Can you work these out from the model? Positions are in its coordinate system, mm. Face numbers are marked on the shaded views. A direction names the side the tool comes from. Give positions to 0.01 mm unless a question says otherwise; leave off trailing zeros. Loops run counter-clockwise (first coordinate to the right, second up) from the corner with the lowest first, then second, coordinate; pieces in that order, holes last. Notation, with made-up numbers: M 37,18.25 L 48,18.25 A28 ccw 48,41.25 Z; hole C 48,-22.5 d4. An arc over 180 degrees is marked long. Use CSV: the item, a comma, the result in double quotes.
from build123d import *

# Parameters (mm, degrees)
RESSALTO_EXTRUS_O1_DEPTH = 22.5
CHANFRO1_SIZE            = 10
CORTE_EXTRUS_O1_REACH    = 324.073
ESBO_O3_W                = 1139.230904301
ESBO_O3_H                = 709.798033895
CORTE_EXTRUS_O5_DEPTH    = 1.5
ESBO_O5_R                = 3
CORTE_EXTRUS_O6_DEPTH    = 322.972048476
CORTE_EXTRUS_O8_DEPTH    = 10


with BuildPart() as part:
    # Esboço1 → Ressalto-extrusão1 (new, symmetric)
    with BuildSketch(Plane.XY):
        with BuildLine():
            Line((-70, 0), (70, 0))
            ThreePointArc((70, 0), (77.071067812, 2.928932188), (80, 10))
            Line((80, 10), (80, 100))
            ThreePointArc((80, 100), (80.93692213, 104.226182617), (83.572123903, 107.660444431))
            Line((83.572123903, 107.660444431), (111.427876097, 131.034195823))
            ThreePointArc((111.427876097, 131.034195823), (114.06307787, 134.468457637), (115, 138.694640254))
            Line((115, 138.694640254), (115, 290))
            ThreePointArc((115, 290), (112.071067812, 297.071067812), (105, 300))
            Line((105, 300), (-105, 300))
            ThreePointArc((-105, 300), (-112.071067812, 297.071067812), (-115, 290))
            Line((-115, 290), (-115, 138.694640254))
            ThreePointArc((-115, 138.694640254), (-114.06307787, 134.468457637), (-111.427876097, 131.034195823))
            Line((-111.427876097, 131.034195823), (-83.572123903, 107.660444431))
            ThreePointArc((-83.572123903, 107.660444431), (-80.93692213, 104.226182617), (-80, 100))
            Line((-80, 100), (-80, 10))
            ThreePointArc((-80, 10), (-77.071067812, 2.928932188), (-70, 0))
        make_face()
        Polygon((-55, 20), (55, 20), (55, 109.793731589), (90, 139.16221868), (90, 280), (-90, 280), (-90, 139.16221868), (-55, 109.793731589), align=None, mode=Mode.SUBTRACT)
    extrude(amount=RESSALTO_EXTRUS_O1_DEPTH, both=True)

    # Chanfro1
    chanfro1_edges = [part.edges().sort_by_distance(p)[0] for p in [
        (114.06307787, 134.468457637, 22.5),
        (115, 214.347320127, 22.5),
        (115, 214.347320127, -22.5),
        (114.06307787, 134.468457637, -22.5),
        (97.5, 119.347320127, -22.5),
        (80.93692213, 104.226182617, -22.5),
        (80, 55, -22.5),
        (77.071067812, 2.928932188, -22.5),
        (0, 0, -22.5),
        (-77.071067812, 2.928932188, -22.5),
        (-80, 55, -22.5),
        (-80.93692213, 104.226182617, -22.5),
        (-97.5, 119.347320127, -22.5),
        (-114.06307787, 134.468457637, -22.5),
        (-115, 214.347320127, -22.5),
        (-112.071067812, 297.071067812, -22.5),
        (0, 300, -22.5),
        (112.071067812, 297.071067812, -22.5),
        (112.071067812, 297.071067812, 22.5),
        (0, 300, 22.5),
        (-112.071067812, 297.071067812, 22.5),
        (-115, 214.347320127, 22.5),
        (-114.06307787, 134.468457637, 22.5),
        (-97.5, 119.347320127, 22.5),
        (-80.93692213, 104.226182617, 22.5),
        (-80, 55, 22.5),
        (-77.071067812, 2.928932188, 22.5),
        (0, 0, 22.5),
        (77.071067812, 2.928932188, 22.5),
        (80, 55, 22.5),
        (80.93692213, 104.226182617, 22.5),
        (97.5, 119.347320127, 22.5),
    ]]
    chamfer(chanfro1_edges, length=CHANFRO1_SIZE - 0.0001)  # a hair under: the kernel refuses the full size

    # Esboço3 → Corte-extrusão1 (cut, up to next)
    with BuildSketch(Plane.XY, mode=Mode.PRIVATE) as corte_extrus_o1_sk1:
        with Locations((-153.157436203, 152.53565808)):
            Rectangle(ESBO_O3_W, ESBO_O3_H)
    corte_extrus_o1_tool1 = extrude(corte_extrus_o1_sk1.sketch, amount=-CORTE_EXTRUS_O1_REACH, mode=Mode.PRIVATE) & part.part
    add(corte_extrus_o1_tool1.solids().sort_by_distance((-153.157436, 152.535658, 0))[0], mode=Mode.SUBTRACT)

    # Esboço4 → Corte-extrusão5 (cut)
    with BuildSketch(Plane.XY.offset(22.5)):
        Polygon((104, 289), (-104, 289), (-104, 139.160947912), (-69, 109.792460821), (-69, 11), (69, 11), (69, 109.792460821), (104, 139.160947912), align=None)
        Polygon((-90, 280), (-90, 139.16221868), (-55, 109.793731589), (-55, 20), (0, 20), (55, 20), (55, 109.793731589), (90, 139.16221868), (90, 280), align=None, mode=Mode.SUBTRACT)
    extrude(amount=-CORTE_EXTRUS_O5_DEPTH, mode=Mode.SUBTRACT)

    # Esboço5 → Corte-extrusão6 (cut, through all)
    with BuildSketch(Plane.XY.offset(21)):
        with Locations((-97, 244)):
            Circle(ESBO_O5_R)
        with Locations((-62, 60.396230411)):
            Circle(ESBO_O5_R)
        with Locations((-97, 282)):
            Circle(ESBO_O5_R)
        with Locations((-62, 18)):
            Circle(ESBO_O5_R)
        with Locations(Location((62, 18, 0), (0, 0, 180))):
            Circle(ESBO_O5_R)
        with Locations(Location((97, 282, 0), (0, 0, 180))):
            Circle(ESBO_O5_R)
        with Locations(Location((62, 60.396230411, 0), (0, 0, 180))):
            Circle(ESBO_O5_R)
        with Locations(Location((97, 244, 0), (0, 0, 180))):
            Circle(ESBO_O5_R)
    extrude(amount=-CORTE_EXTRUS_O6_DEPTH, mode=Mode.SUBTRACT)

    # Esboço7 → Corte-extrusão8 (cut)
    with BuildSketch(Plane(origin=(0, 0, 0), x_dir=(-1, 0, 0), z_dir=(0, 0, -1))):
        Polygon((-96.223646947, 288.060191195), (-101.860103, 285.702437064), (-102.636456053, 279.642245869), (-97.776353053, 275.939808805), (-92.139897, 278.297562936), (-91.363543947, 284.357754131), align=None)
        Polygon((-96.739022153, 247.917298035), (-100.261990689, 246.184662463), (-100.522968536, 242.267364427), (-97.260977847, 240.082701965), (-93.738009311, 241.815337537), (-93.477031464, 245.732635573), align=None)
        Polygon((-62, 64.322212241), (-65.4, 62.359221326), (-65.4, 58.433239495), (-62, 56.47024858), (-58.6, 58.433239495), (-58.6, 62.359221326), align=None)
        Polygon((-62, 19.92598183), (-63.667949192, 18.962990915), (-63.667949192, 17.037009085), (-62, 16.07401817), (-60.332050808, 17.037009085), (-60.332050808, 18.962990915), align=None)
        Polygon((62.727937948, 19.561318936), (61.011827112, 19.411072223), (60.283889164, 17.849753287), (61.272062052, 16.438681064), (62.988172888, 16.588927777), (63.716110836, 18.150246713), align=None)
        Polygon((62, 64.322212241), (58.6, 62.359221326), (58.6, 58.433239495), (62, 56.47024858), (65.4, 58.433239495), (65.4, 62.359221326), align=None)
        Polygon((97, 247.92598183), (93.6, 245.962990915), (93.6, 242.037009085), (97, 240.07401817), (100.4, 242.037009085), (100.4, 245.962990915), align=None)
        Polygon((97, 287.92598183), (91.867949192, 284.962990915), (91.867949192, 279.037009085), (97, 276.07401817), (102.132050808, 279.037009085), (102.132050808, 284.962990915), align=None)
    extrude(amount=-CORTE_EXTRUS_O8_DEPTH, mode=Mode.SUBTRACT)


solid = part.part
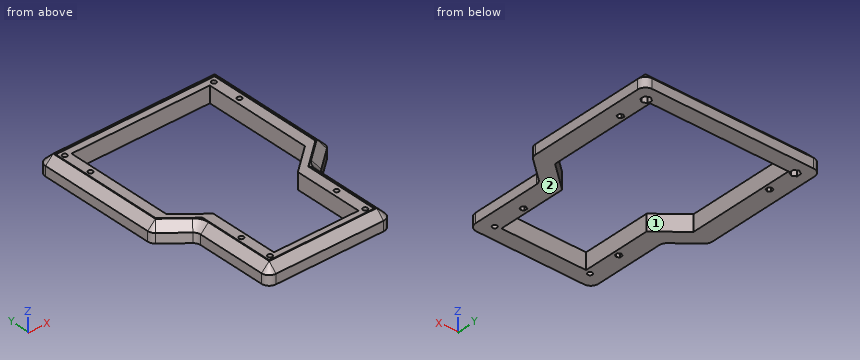
Q1. I'm going to push flat-ended pins straight in: P1, Ø3.5, axis at x = 97, y = 244, coming from the -Z side; P2, Ø9.5, axis at x = 62, y = 18, coming from the -Z side; P3, Ø1.2, axis at x = -19.5, z = 22, coming from the +Y side; P4, Ø8, axis at x = -55.5, z = 19.5, coming from the -Y side. Where does each tip first touch, or does it pass through?
Model answer:
P1,"through"
P2,"z = 0"
P3,"y = 291.1"
P4,"y = 3"
Q2. I want a section at A-A, the plane x = -41. Please give me the cut outline in (y, z).
Model answer:
outline,"M 0,0 L 20,0 L 20,21 L 11,21 L 11,22.5 L 10,22.5 L 0,12.5 Z; M 280,0 L 300,0 L 300,12.5 L 290,22.5 L 289,22.5 L 289,21 L 280,21 Z"
Q3. I want a section at B-B, the plane y = 200. Please give me the cut outline in (x, z), then the cut area to 3 significant figures.
Model answer:
outline,"M -115,0 L -90,0 L -90,21 L -104,21 L -104,22.5 L -105,22.5 L -115,12.5 Z; M 90,0 L 115,0 L 115,12.5 L 105,22.5 L 104,22.5 L 104,21 L 90,21 Z"
area,"983 mm2"
Q4. For the marked faces 1 and 2, which set-ups out of +Z, -Z, +X, -X, +Y, -Y let a thin tool reach every point of the face, with its end or its side?
Model answer:
face 1,"+Z, -Z"
face 2,"-Z, +X, -X, +Y, -Y"
Q5. Please list where these lines run through material, in increasing order: L1, parallel to X at y = 245.5, z = 1.75; L2, parallel to X at y = 200, z = 4; L3, parallel to X at y = 282, z = 13. Write a range as from..to.
Model answer:
L1,"-115..-100.4, -93.6..-90, 90..93.49, 100.31..115"
L2,"-115..-90, 90..115"
L3,"-114.5..-100, -94..94, 100..114.5"
